Input: part model. Units: mm. Frame: model coordinates. A direction names the side the tool comes from. Give positions to 0.01 mm unless a question says otherwise; leave off trailing zeros. Order: outer loops, then holes, each group sorted by start corner. A loop starts at its lowest first (then second) coordinate and runs counter-clockwise, first axis right, second up. Notation, with made-up numbers: M 44,-28.75 L 68,-28.75 A14 ccw 68,-23.75 Z; hole C 41,-18.5 d9. An arc over 180 degrees is marked long. Use a Markdown table: item, result.
from build123d import *

# Parameters (mm, degrees)
SKETCH1_W               = 156
SKETCH1_H               = 25
SKETCH1_R               = 2.5
SKETCH1_R_2             = 3
BOSS_EXTRUDE1_DEPTH     = 6
FILLET1_R               = 2.5
SKETCH2_R               = 2
CUT_EXTRUDE1_DEPTH      = 10
LPATTERN1_COUNT         = 6
LPATTERN1_PITCH         = 26
MIRROR1_COPY_1_SKETCH_R = 2
MIRROR1_COPY_1_DEPTH    = 10
MIRROR1_COPY_2_SKETCH_R = 2
MIRROR1_COPY_2_DEPTH    = 10
MIRROR1_COPY_3_SKETCH_R = 2
MIRROR1_COPY_3_DEPTH    = 10
MIRROR1_COPY_4_SKETCH_R = 2
MIRROR1_COPY_4_DEPTH    = 10
MIRROR1_COPY_5_SKETCH_R = 2
MIRROR1_COPY_5_DEPTH    = 10


with BuildPart() as part:
    # Sketch1 → Boss-Extrude1 (new, symmetric)
    with BuildSketch(Plane(origin=(0, 0, 0), x_dir=(1, 0, 0), z_dir=(0, 1, 0))):
        Rectangle(SKETCH1_W, SKETCH1_H)
        with Locations(Location((0, 0, 0), (0, 0, 270))):
            Circle(SKETCH1_R, mode=Mode.SUBTRACT)
        with Locations(Location((-56, -3, 0), (0, 0, 270))):
            Circle(SKETCH1_R_2, mode=Mode.SUBTRACT)
        with Locations(Location((-26, -3, 0), (0, 0, 270))):
            Circle(SKETCH1_R_2, mode=Mode.SUBTRACT)
        with Locations(Location((56, -3, 0), (0, 0, 90))):
            Circle(SKETCH1_R_2, mode=Mode.SUBTRACT)
        with Locations(Location((26, -3, 0), (0, 0, 90))):
            Circle(SKETCH1_R_2, mode=Mode.SUBTRACT)
    extrude(amount=BOSS_EXTRUDE1_DEPTH, both=True)

    # Fillet1
    fillet1_edges = [part.edges().sort_by_distance(p)[0] for p in [
        (-78, 6, 0),
        (78, 6, 0),
        (-78, -6, 0),
        (78, -6, 0),
    ]]
    fillet(fillet1_edges, radius=FILLET1_R)

    # Sketch2 → Cut-Extrude1 (cut)
    with BuildSketch(Plane.XY.offset(12.5)):
        with Locations((-65, 0)):
            Circle(SKETCH2_R)
    cut_extrude1 = extrude(amount=-CUT_EXTRUDE1_DEPTH, mode=Mode.SUBTRACT)

    # LPattern1: Cut-Extrude1 ×6
    with Locations(*[(i * LPATTERN1_PITCH, 0, 0) for i in range(1, LPATTERN1_COUNT)]):
        add(cut_extrude1, mode=Mode.SUBTRACT)

    # Mirror1: Cut-Extrude1 across plane
    add(cut_extrude1.mirror(Plane.XY), mode=Mode.SUBTRACT)

    # Mirror1 copy 1 sketch → Mirror1 copy 1 (cut)
    with BuildSketch(Plane(origin=(26, 0, -12.5), x_dir=(1, 0, 0), z_dir=(0, 0, -1))):
        with Locations((-65, 0)):
            Circle(MIRROR1_COPY_1_SKETCH_R)
    extrude(amount=-MIRROR1_COPY_1_DEPTH, mode=Mode.SUBTRACT)

    # Mirror1 copy 2 sketch → Mirror1 copy 2 (cut)
    with BuildSketch(Plane(origin=(52, 0, -12.5), x_dir=(1, 0, 0), z_dir=(0, 0, -1))):
        with Locations((-65, 0)):
            Circle(MIRROR1_COPY_2_SKETCH_R)
    extrude(amount=-MIRROR1_COPY_2_DEPTH, mode=Mode.SUBTRACT)

    # Mirror1 copy 3 sketch → Mirror1 copy 3 (cut)
    with BuildSketch(Plane(origin=(78, 0, -12.5), x_dir=(1, 0, 0), z_dir=(0, 0, -1))):
        with Locations((-65, 0)):
            Circle(MIRROR1_COPY_3_SKETCH_R)
    extrude(amount=-MIRROR1_COPY_3_DEPTH, mode=Mode.SUBTRACT)

    # Mirror1 copy 4 sketch → Mirror1 copy 4 (cut)
    with BuildSketch(Plane(origin=(104, 0, -12.5), x_dir=(1, 0, 0), z_dir=(0, 0, -1))):
        with Locations((-65, 0)):
            Circle(MIRROR1_COPY_4_SKETCH_R)
    extrude(amount=-MIRROR1_COPY_4_DEPTH, mode=Mode.SUBTRACT)

    # Mirror1 copy 5 sketch → Mirror1 copy 5 (cut)
    with BuildSketch(Plane(origin=(130, 0, -12.5), x_dir=(1, 0, 0), z_dir=(0, 0, -1))):
        with Locations((-65, 0)):
            Circle(MIRROR1_COPY_5_SKETCH_R)
    extrude(amount=-MIRROR1_COPY_5_DEPTH, mode=Mode.SUBTRACT)


solid = part.part
1) Cut plane A-A on x = -26. Return loops of the section in (y, z), and give its area (3 significant figures).
Response values:
| item | result |
|---|---|
| outline | M -6,-12.5 L 6,-12.5 L 6,0 L -6,0 Z; M -6,6 L 6,6 L 6,12.5 L -6,12.5 Z |
| area | 228 mm² |
2) Material intervals for line 1 (X direction, y = -2.5, z = 3); line 2 (X direction, y = -2, z = 2.25); line 3 (Z direction, x = 26, y = -1.25), sorted ascending. Write a range as from..to.
Response values:
| item | result |
|---|---|
| line 1 | x = -78..-59, -53..-29, -23..23, 29..53, 59..78 |
| line 2 | x = -78..-58.9, -53.1..-28.9, -23.1..-1.09, 1.09..23.1, 28.9..53.1, 58.9..78 |
| line 3 | z = -12.5..0, 6..12.5 |
3) Cut plane B-B on z = 10.25. Return loops of the section in (x, y).
Response values:
| item | result |
|---|---|
| outline | M -78,-3.5 A2.5 ccw -75.5,-6 L 75.5,-6 A2.5 ccw 78,-3.5 L 78,3.5 A2.5 ccw 75.5,6 L -75.5,6 A2.5 ccw -78,3.5 Z; hole C -65,0 d4; hole C -39,0 d4; hole C -13,0 d4; hole C 13,0 d4; hole C 39,0 d4; hole C 65,0 d4 |
4) Mould query, pull axis Z, two halves, no side actions, for faces 1 (the face through (39, 0, -2.5)), 2 (the face through (-2.44, -0.08, -0.54)), 3 (the face through (77.248, 5.287, -0.175)). Classes: released by +Z, released by -Z, zero draft, split by the parting line, or undercut.
Response values:
| item | result |
|---|---|
| face 1 | released by -Z |
| face 2 | undercut |
| face 3 | zero draft |
5) First-contact query: pin 1 Ø4.5 at (x, y) = (-66, -1) entering from -Z; pin 2 Ø2.5 at (x, y) = (39, 0) entering from -Z; pin 3 Ø3 at (x, y) = (13, 0) entering from +Z. Flat tips, straight axial feed; report the tip coordinate or a pass-through.
Response values:
| item | result |
|---|---|
| pin 1 | stops at z = -12.5 |
| pin 2 | stops at z = -2.5 |
| pin 3 | stops at z = 2.5 |
6) Reachability of faces 4 (the face through (-65, 0, 2.5)), 5 (the face through (-13, 0, -2.5)), 6 (the face through (-1, 6, -3)) from +Z, -Z, +X, -X, +Y, -Y: full face, straight path, thin tool, end or side. Return the list, or none.
Response values:
| item | result |
|---|---|
| face 4 | +Z |
| face 5 | -Z |
| face 6 | +Z, -Z, +X, -X, +Y |
